from build123d import *

# Parameters (mm, degrees)
SKETCH_1_W          = 50
SKETCH_1_H          = 37.5
SKETCH_1_R          = 1.5
SKETCH_1_R_2        = 1
SKETCH_1_W_2        = 24
SKETCH_1_H_2        = 14
EXTRUDE_1_DEPTH     = 3
FILLET_1_R          = 5
SKETCH_2_R          = 2
CUT_EXTRUDE_1_DEPTH = 10


with BuildPart() as part:
    # 草图1 → 凸台-拉伸1 (new body)
    with BuildSketch(Plane(origin=(0, 0, 0), x_dir=(1, 0, 0), z_dir=(0, 1, 0))):
        Rectangle(SKETCH_1_W, SKETCH_1_H)
        with Locations(Location((4, -11.75, 0), (0, 0, 270))):
            Circle(SKETCH_1_R, mode=Mode.SUBTRACT)
        with Locations(Location((-4, -11.75, 0), (0, 0, 90))):
            Circle(SKETCH_1_R, mode=Mode.SUBTRACT)
        with Locations(Location((7.29, 3.75, 0), (0, 0, 270))):
            Circle(SKETCH_1_R_2, mode=Mode.SUBTRACT)
        with Locations(Location((-20.51, 3.75, 0), (0, 0, 90))):
            Circle(SKETCH_1_R_2, mode=Mode.SUBTRACT)
        with Locations((-6.61, 3.75)):
            Rectangle(SKETCH_1_W_2, SKETCH_1_H_2, mode=Mode.SUBTRACT)
    extrude(amount=EXTRUDE_1_DEPTH)

    # 圆角1
    fillet_1_edges = [part.edges().sort_by_distance(p)[0] for p in [
        (25, 1.5, 18.75),
        (-25, 1.5, 18.75),
        (-25, 1.5, -18.75),
        (25, 1.5, -18.75),
    ]]
    fillet(fillet_1_edges, radius=FILLET_1_R)

    # 草图2 → 切除-拉伸1 (cut)
    with BuildSketch(Plane(origin=(0, 3, 0), x_dir=(1, 0, 0), z_dir=(0, 1, 0))):
        with Locations(Location((12.5, 3.75, 0), (0, 0, 270))):
            Circle(SKETCH_2_R)
    extrude(amount=-CUT_EXTRUDE_1_DEPTH, mode=Mode.SUBTRACT)


solid = part.part
Can you work these out from the model? Positions are in its coordinate system, mm. A direction names the side the tool comes from. Give positions to 0.01 mm unless a question says otherwise; leave off trailing zeros. Order: outer loops, then holes, each group sorted by start corner. A loop starts at its lowest first (then second) coordinate and runs counter-clockwise, first axis right, second up. Notation, with made-up numbers: M 57.5,0 L 64.5,0 A15 cw 64.5,19 Z; hole C 24.25,75.25 d2. An arc over 180 degrees is marked long. Use a Markdown table: item, result. Add a question column.
Item 1: Suppose I cut it at C-C (z = -3.75). List the corners of the cut face in (x, y) for me, then the cut area to 3 significant figures.
Item 2: Suppose I cut it at B-B (z = 11.75). List the corners of the cut face in (x, y) for me, then the cut area to 3 significant figures.
Item 3: If I drill on L1, parallel to X at y = 1.45, z = -3.75; L2, parallel to Z at x = -2, y = 2.6; L3, parallel to X at y = 2, z = 11.75, over which ranges is the centre line in solid material (lowest first)? Write a range as [from, to].
Item 4: Suppose I cut it at A-A (x = 4). List the corners of the cut face in (y, z) for me, then the cut area to 3 significant figures.
Item 5: Suppose I cut it at D-D (y = 2.55). List the corners of the cut face in (x, z) for me, then the cut area to 3 significant figures.
Item 6: We'd pull the mould along Z, two halves only. Please class faces 3 (the flat face through (25, 1, 0)), 4 (the cylindrical face through (6.68, 1.48, -4.54)), 5 (the flat face through (0, 1, 18.75)): +Z half, -Z half, draft (parallel to the pull), parting line (faces both ways), or undercut.
Item 7: For faces 1 (the cylindrical face through (23.5, 1.52, -17.32)), 2 (the flat face through (-18.61, 1, -4)), which set-ups out of +Z, -Z, +X, -X, +Y, -Y let a thin tool reach every point of the face, with its end or its side?
Answer sheet:
| question | item | result |
|---|---|---|
| 1 | outline | M -25,0 L -21.51,0 L -21.51,3 L -25,3 Z; M -19.51,0 L -18.61,0 L -18.61,3 L -19.51,3 Z; M 5.39,0 L 6.29,0 L 6.29,3 L 5.39,3 Z; M 8.29,0 L 10.5,0 L 10.5,3 L 8.29,3 Z; M 14.5,0 L 25,0 L 25,3 L 14.5,3 Z |
| 1 | area | 54.0 mm² |
| 2 | outline | M -25,0 L -5.5,0 L -5.5,3 L -25,3 Z; M -2.5,0 L 2.5,0 L 2.5,3 L -2.5,3 Z; M 5.5,0 L 25,0 L 25,3 L 5.5,3 Z |
| 2 | area | 132 mm² |
| 3 | L1 | x = [-25, -21.51], [-19.51, -18.61], [5.39, 6.29], [8.29, 10.5], [14.5, 25] |
| 3 | L2 | z = [-18.75, -10.75], [3.25, 18.75] |
| 3 | L3 | x = [-25, -5.5], [-2.5, 2.5], [5.5, 25] |
| 4 | outline | M 0,-18.75 L 3,-18.75 L 3,-10.75 L 0,-10.75 Z; M 0,3.25 L 3,3.25 L 3,10.25 L 0,10.25 Z; M 0,13.25 L 3,13.25 L 3,18.75 L 0,18.75 Z |
| 4 | area | 61.5 mm² |
| 5 | outline | M -25,-13.75 A5 ccw -20,-18.75 L 20,-18.75 A5 ccw 25,-13.75 L 25,13.75 A5 ccw 20,18.75 L -20,18.75 A5 ccw -25,13.75 Z; hole C -20.51,-3.75 d2; hole M -18.61,-10.75 L 5.39,-10.75 L 5.39,3.25 L -18.61,3.25 Z; hole C -4,11.75 d3; hole C 4,11.75 d3; hole C 7.29,-3.75 d2; hole C 12.5,-3.75 d4 |
| 5 | area | 1,480 mm² |
| 6 | face 3 | draft |
| 6 | face 4 | undercut |
| 6 | face 5 | +Z half |
| 7 | face 1 | -Z, +X, +Y, -Y |
| 7 | face 2 | +Y, -Y |
